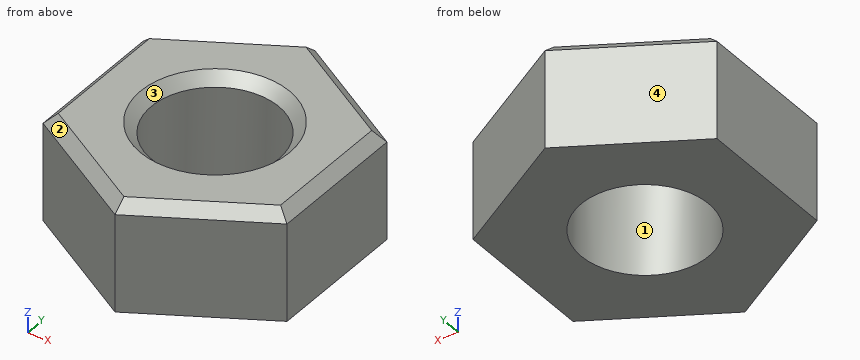
from build123d import *

# Parameters (mm, degrees)
SKETCH1_R           = 2.35
BOSS_EXTRUDE1_DEPTH = 4
CHAMFER1_SIZE       = 0.4


with BuildPart() as part:
    # Sketch1 → Boss-Extrude1 (new body)
    with BuildSketch(Plane.XY):
        Polygon((4.5, -2.598076211), (4.5, 2.598076211), (0, 5.196152423), (-4.5, 2.598076211), (-4.5, -2.598076211), (0, -5.196152423), align=None)
        Circle(SKETCH1_R, mode=Mode.SUBTRACT)
    extrude(amount=BOSS_EXTRUDE1_DEPTH)

    # Chamfer1
    chamfer1_edges = [part.edges().sort_by_distance(p)[0] for p in [
        (2.25, 3.897114317, 4),
        (-2.25, 3.897114317, 4),
        (-2.35, 0, 4),
        (-4.5, 0, 4),
        (-2.25, -3.897114317, 4),
        (2.25, -3.897114317, 4),
        (4.5, 0, 4),
    ]]
    chamfer(chamfer1_edges, length=CHAMFER1_SIZE)


solid = part.part
Model file for the job. Use its own axes, mm. Face numbers are marked on the shaded views. Coordinates: 2 decimals unless noted, no trailing zeros. Loops run counter-clockwise (first coordinate to the right, second up) from the corner with the lowest first, then second, coordinate; pieces in that order, holes last. Notation, with made-up numbers: (89, -16.5) -> (133, -16.5) arc R29 ccw to (133, 4.5) -> close; hole circle Ø10 at (84, -37). An arc over 180 degrees is marked (long way). Use one line per item in the form item = value. Start each with the question number.
(1) Pull direction Y, two halves, no side cores. Call the marked faces 1, 2, 3 and 4: pulls with the +Y half, pulls with the -Y half, needs draft (parallel to the pull), parting line crosses it, or undercut.
(2) Cut at D-D on x = -3.25. Give the cut face in (y, z), and give its area (3 significant figures).
(3) Flat gauge pins, fed straight in: pin 1 (1 mm diameter, centred on y = 4, z = 1.5, fed in from +X); pin 2 (1 mm diameter, centred on x = 1.5, z = 1, fed in from +Y). Where does each tip first touch, or does it go through?
(4) Cut at B-B on z = 1.1. Give the cut face in (x, y), and give its area (3 significant figures).
(5) Cut at A-A on y = 0. Give the cut face in (x, z).
(6) Cut at C-C on y = -3.25. Give the cut face in (x, z).
(7) Probe probe 1 along Y at (x, z) = (0.5, 3.1); probe 2 along Y at (x, z) = (-2, 1.15); probe 3 along X at (y, z) = (-0.75, 3.75). List the from-to ranges inside material, lowest first. Write a range as from..to.
Values:
q1.face_1 = undercut
q1.face_2 = pulls with the -Y half
q1.face_3 = undercut
q1.face_4 = pulls with the +Y half
q2.outline = (-3.32, 0) -> (3.32, 0) -> (3.32, 3.6) -> (2.86, 4) -> (-2.86, 4) -> (-3.32, 3.6) -> close
q2.area = 26.4 mm2
q3.pin_1 = 2.94
q3.pin_2 = 4.62
q4.outline = (-4.5, -2.6) -> (0, -5.2) -> (4.5, -2.6) -> (4.5, 2.6) -> (0, 5.2) -> (-4.5, 2.6) -> close; hole circle Ø4.7 at (0, 0)
q4.area = 52.8 mm2
q5.outline = (-4.5, 0) -> (-2.35, 0) -> (-2.35, 3.6) -> (-2.75, 4) -> (-4.1, 4) -> (-4.5, 3.6) -> close; (2.35, 0) -> (4.5, 0) -> (4.5, 3.6) -> (4.1, 4) -> (2.75, 4) -> (2.35, 3.6) -> close
q6.outline = (-3.37, 0) -> (3.37, 0) -> (3.37, 3.6) -> (2.57, 4) -> (-2.57, 4) -> (-3.37, 3.6) -> close
q7.probe_1 = -4.91..-2.3, 2.3..4.91
q7.probe_2 = -4.04..-1.23, 1.23..4.04
q7.probe_3 = -4.35..-2.38, 2.38..4.35
